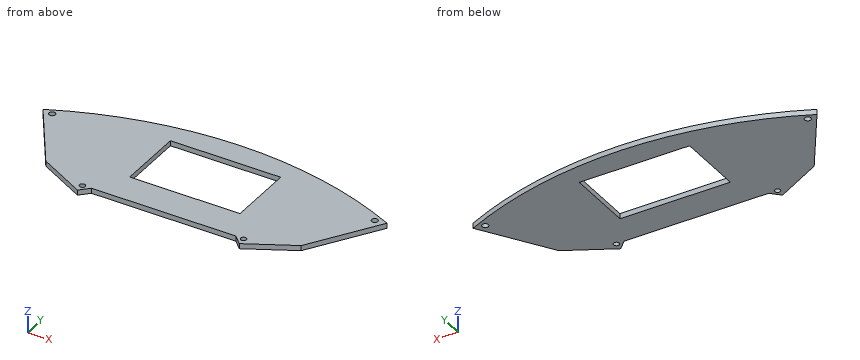
```python
from build123d import *

# Parameters (mm, degrees)
BOSS_EXTRUDE1_DEPTH = 4
SKETCH2_W           = 85
SKETCH2_H           = 51.5
CUT_EXTRUDE1_DEPTH  = 20
CUT_EXTRUDE3_START  = 10
SKETCH3_R           = 2.404549827
SKETCH3_R_2         = 2.15
CUT_EXTRUDE3_DEPTH  = 20


with BuildPart() as part:
    # Sketch1 → Boss-Extrude1 (new body)
    with BuildSketch(Plane.XY):
        with BuildLine():
            Line((-54.022988506, -46.729885057), (-60.700936328, -53.40783288))
            Line((-60.700936328, -53.40783288), (-96.723977713, -34.253129761))
            Line((-96.723977713, -34.253129761), (-130.872988506, 18.270114943))
            ThreePointArc((-130.872988506, 18.270114943), (1.627011494, 48.270114943), (134.127011494, 18.270114943))
            Line((134.127011494, 18.270114943), (99.978000701, -34.253129761))
            Line((99.978000701, -34.253129761), (63.954959317, -53.40783288))
            Line((63.954959317, -53.40783288), (57.277011494, -46.729885057))
            Line((57.277011494, -46.729885057), (-54.022988506, -46.729885057))
        make_face()
    extrude(amount=BOSS_EXTRUDE1_DEPTH)

    # Sketch2 → Cut-Extrude1 (cut)
    with BuildSketch(Plane.XY):
        with Locations((2.977011494, 3.662316168)):
            Rectangle(SKETCH2_W, SKETCH2_H)
    extrude(amount=CUT_EXTRUDE1_DEPTH, mode=Mode.SUBTRACT)

    # Sketch3 → Cut-Extrude3 (cut)
    with BuildSketch(Plane.XY.offset(CUT_EXTRUDE3_START)):
        with Locations(Location((-122.881880972, 16.804537187, 0), (0, 0, 180))):
            Circle(SKETCH3_R)
        with Locations(Location((-60.728139954, -47.058565961, 0), (0, 0, 180))):
            Circle(SKETCH3_R_2)
        with Locations(Location((63.420208839, -47.058565961, 0), (0, 0, 180))):
            Circle(SKETCH3_R_2)
        with Locations(Location((125.573949857, 16.804537187, 0), (0, 0, 180))):
            Circle(SKETCH3_R)
    extrude(amount=-CUT_EXTRUDE3_DEPTH, mode=Mode.SUBTRACT)


solid = part.part
```
Can you work these out from the model? Positions are in its coordinate system, mm. Give positions to 0.01 mm unless a question says otherwise; leave off trailing zeros. Write each loop counter-clockwise with the first axis right and the second up, starting at its lowest first coordinate (ties: lowest second). Pieces come first, ordered by that corner, then holes. Notation, with made-up numbers: (-3.75, -15) -> (14.25, -15) arc R34 cw to (14.25, 16) -> close; hole circle Ø8 at (-23.75, -2.75). An arc over 180 degrees is marked (long way). One line per item, written item: value.
Q1. Imagine slicing it at B-B on y = 12. Please give me the cut outline in (x, z), and give its area (3 significant figures).
Results found:
outline: (-126.8, 0) -> (-39.52, 0) -> (-39.52, 4) -> (-126.8, 4) -> close; (45.48, 0) -> (130.05, 0) -> (130.05, 4) -> (45.48, 4) -> close
area: 687 mm^2
Q2. Please list where these lines run through material, in increasing order: line 1 (X direction, y = -48.5, z = 1.15); line 2 (X direction, y = -46.5, z = 1.95); line 3 (Y direction, x = -2, z = 2.3). Write a range as [from, to].
Results found:
line 1: x = [-69.93, -62.32], [-59.13, -55.79], [59.05, 61.82], [65.02, 73.18]
line 2: x = [-73.69, -62.8], [-58.65, 61.34], [65.5, 76.95]
line 3: y = [-46.73, -22.09], [29.41, 48.25]
Q3. Imagine slicing it at C-C on z = 1.4. Please give me the cut outline in (x, y).
Results found:
outline: (-130.87, 18.27) -> (-96.72, -34.25) -> (-60.7, -53.41) -> (-54.02, -46.73) -> (57.28, -46.73) -> (63.95, -53.41) -> (99.98, -34.25) -> (134.13, 18.27) arc R307.6 ccw to start; hole circle Ø4.81 at (-122.88, 16.8); hole circle Ø4.3 at (-60.73, -47.06); hole (-39.52, -22.09) -> (45.48, -22.09) -> (45.48, 29.41) -> (-39.52, 29.41) -> close; hole circle Ø4.3 at (63.42, -47.06); hole circle Ø4.81 at (125.57, 16.8)
Q4. For P1, Ø3, axis at x = 125.57, y = 16.8, coming from the +Z side; P2, Ø5, axis at x = 63.42, y = -47.06, coming from the -Z side; P3, Ø2, axis at x = 6.5, z = 1.5, coming from the -Y side; P4, Ø2, axis at y = 4.5, z = 1.5, coming from the -X side, each with a flat end and sliding along its axis, tell me the tip position at first contact or that it passes through.
Results found:
P1: passes through
P2: stops at z = 0
P3: stops at y = -46.73
P4: stops at x = -122.57
Q5. Imagine slicing it at D-D on x = 113.5. Please give me the cut outline in (y, z), and give its area (3 significant figures).
Results found:
outline: (-13.46, 0) -> (27.21, 0) -> (27.21, 4) -> (-13.46, 4) -> close
area: 163 mm^2
Q6. Imagine slicing it at A-A on x = -19. Please give me the cut outline in (y, z).
Results found:
outline: (-46.73, 0) -> (-22.09, 0) -> (-22.09, 4) -> (-46.73, 4) -> close; (29.41, 0) -> (47.58, 0) -> (47.58, 4) -> (29.41, 4) -> close
